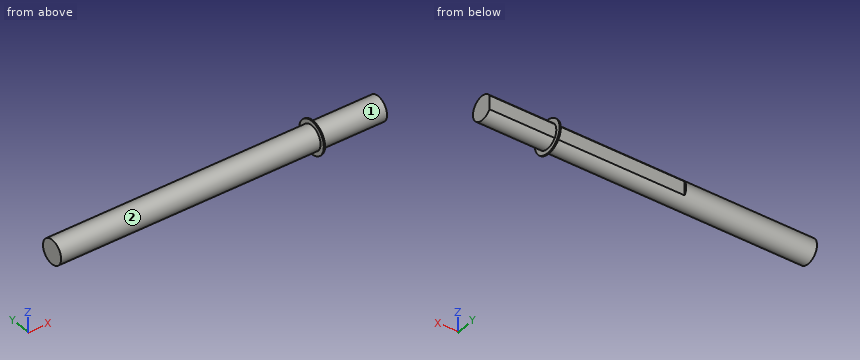
```python
from build123d import *

# Parameters (mm, degrees)
ENL_V_START             = -45.5
ENL_V_MAT_EXTRU_1_DEPTH = 45.5


with BuildPart() as part:
    # Esquisse1 → Révolution1 (revolve)
    with BuildSketch(Plane.XY, mode=Mode.PRIVATE) as r_volution1_sk:
        Polygon((60.8, 2.8), (60.8, 3.8), (60.5, 3.8), (60.5, 2.8), (0, 2.8), (0, 0), (76, 0), (76, 2.8), align=None)
    revolve(r_volution1_sk.sketch.rotate(Axis((0, 0, 0), (1, 0, 0)), 90), axis=Axis((0, 0, 0), (1, 0, 0)))

    # Esquisse2 → Enlèv. mat.-Extru.1 (cut)
    with BuildSketch(Plane(origin=(76, 0, 0), x_dir=(0, 0, -1), z_dir=(1, 0, 0)).offset(ENL_V_START)):
        with BuildLine():
            Line((-1.596871942, 2.3), (1.596871942, 2.3))
            ThreePointArc((1.596871942, 2.3), (0, 2.8), (-1.596871942, 2.3))
        make_face()
    extrude(amount=ENL_V_MAT_EXTRU_1_DEPTH, mode=Mode.SUBTRACT)


solid = part.part
```
The listing builds one solid part. Answer for the finished solid, in the listing's coordinates (mm). Face numbers are marked on the shaded views. A direction names the side the tool comes from. Coordinates: 2 decimals unless noted, no trailing zeros. Loops run counter-clockwise (first coordinate to the right, second up) from the corner with the lowest first, then second, coordinate; pieces in that order, holes last. Notation, with made-up numbers: (-15, 5.5) -> (2, 5.5) arc R5 cw to (2, 13.5) -> close; hole circle Ø9 at (-28.5, 18.25). An arc over 180 degrees is marked (long way). Use one line per item in the form item = value. Start each with the question number.
Item 1: Flat-ended cylindrical pins translate along their axes: pin 1 Ø4 at (x, y) = (62.5, -2.5) entering from +Z; pin 2 Ø3 at (x, z) = (43.5, -1.5) entering from +Y; pin 3 Ø3 at (x, z) = (28.5, -1.5) entering from -Y. Find the tip coordinate at first contact, or state that the pin passes through.
Item 2: The part is cut by section C-C on x = 53.5. Determine the outline of the cut face in (y, z), then the cut area to 3 significant figures.
Item 3: A tool of negligible diameter and unlimited length cuts with its end or side. For the marked faces 1 and 2, from which of +Z, -Z, +X, -X, +Y, -Y can it reach the whole face along a straight path? Write none if from no direction.
Item 4: Consider L1, parallel to X at y = 3, z = -1; L2, parallel to X at y = 2.5, z = 1; L3, parallel to Y at x = 24, z = -2. Determine where each line is inside the solid, lowest interval first. Write a range as [from, to].
Item 5: The part is cut by section A-A on z = 0. Determine the outline of the cut face in (x, y).
Item 6: The part is cut by section B-B on y = 0. Determine the outline of the cut face in (x, z).
Item 7: The part is cut by section D-D on x = 14.5. Determine the outline of the cut face in (y, z), then the cut area to 3 significant figures.
Answer key:
q1.pin_1 = 3.51
q1.pin_2 = 2.3
q1.pin_3 = -2.8
q2.outline = (2.3, -1.6) -> (2.3, 1.6) arc R2.8 ccw (long way) to start
q2.area = 23.5 mm2
q3.face_1 = +X
q3.face_2 = -X
q4.L1 = [60.5, 60.8]
q4.L2 = [0, 30.5]
q4.L3 = [-1.96, 1.96]
q5.outline = (0, -2.8) -> (60.5, -2.8) -> (60.5, -3.8) -> (60.8, -3.8) -> (60.8, -2.8) -> (76, -2.8) -> (76, 2.3) -> (30.5, 2.3) -> (30.5, 2.8) -> (0, 2.8) -> close; (60.5, 2.8) -> (60.8, 2.8) -> (60.8, 3.8) -> (60.5, 3.8) -> close
q6.outline = (0, -2.8) -> (60.5, -2.8) -> (60.5, -3.8) -> (60.8, -3.8) -> (60.8, -2.8) -> (76, -2.8) -> (76, 2.8) -> (60.8, 2.8) -> (60.8, 3.8) -> (60.5, 3.8) -> (60.5, 2.8) -> (0, 2.8) -> close
q7.outline = circle Ø5.6 at (0, 0)
q7.area = 24.6 mm2
